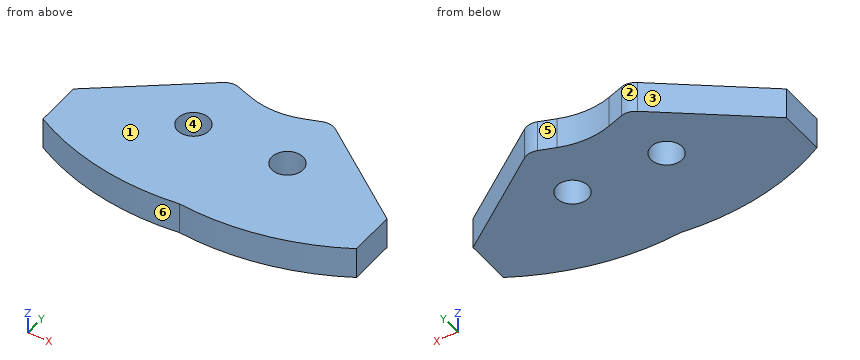
from build123d import *

# Parameters (mm, degrees)
SZKIC1_R                    = 5
DODANIE_WYCI_GNI_CIE1_DEPTH = 10


with BuildPart() as part:
    # Szkic1 → Dodanie-wyciągnięcie1 (new body)
    with BuildSketch(Plane.XY):
        with BuildLine():
            Line((0, 10), (0, 25))
            Line((0, 25), (31.999991312, 49.000008999))
            ThreePointArc((31.999991312, 49.000008999), (34.24374996, 49.942489803), (36.666669828, 49.714055442))
            Line((36.666669828, 49.714055442), (41.666653651, 47.946291102))
            ThreePointArc((41.666653651, 47.946291102), (50, 46.51651254), (58.333346349, 47.946291102))
            Line((58.333346349, 47.946291102), (63.333330172, 49.714055442))
            ThreePointArc((63.333330172, 49.714055442), (65.75625004, 49.942489803), (68.000008688, 49.000008999))
            Line((68.000008688, 49.000008999), (100, 25))
            Line((100, 25), (100, 10))
            ThreePointArc((100, 10), (75.784613824, 1.076930879), (50, 0))
            ThreePointArc((50, 0), (24.215386176, 1.076930879), (0, 10))
        make_face()
        with Locations((35, 30)):
            Circle(SZKIC1_R, mode=Mode.SUBTRACT)
        with Locations(Location((65, 30, 0), (0, 0, 180))):
            Circle(SZKIC1_R, mode=Mode.SUBTRACT)
    extrude(amount=DODANIE_WYCI_GNI_CIE1_DEPTH)


solid = part.part
Here's how the part is built. I have some questions about the finished solid (model axes, mm). Face numbers are marked on the shaded views. A direction names the side the tool comes from. Round coordinates to 2 decimals unless told otherwise and drop trailing zeros. Write each loop counter-clockwise with the first axis right and the second up, starting at its lowest first coordinate (ties: lowest second). Pieces come first, ordered by that corner, then holes. Notation, with made-up numbers: (9.5, 4) -> (26.5, 4) arc R35 ccw to (26.5, 40) -> close; hole circle Ø6 at (12.25, -30). An arc over 180 degrees is marked (long way). One line per item, written item: value.
1) Suppose I cut it at A-A on x = 38. List the corners of the cut face in (y, z) for me.
Filled sheet:
outline: (-0.5, 0) -> (26, 0) -> (26, 10) -> (-0.5, 10) -> close; (34, 0) -> (49.24, 0) -> (49.24, 10) -> (34, 10) -> close
2) Suppose I cut it at B-B on z = 4.75. List the corners of the cut face in (x, y) for me, plus the area to 3 significant figures.
Filled sheet:
outline: (0, 10) arc R83.23 ccw to (50, 0) arc R83.23 ccw to (100, 10) -> (100, 25) -> (68, 49) arc R5 ccw to (63.33, 49.71) -> (58.33, 47.95) arc R25 cw to (41.67, 47.95) -> (36.67, 49.71) arc R5 ccw to (32, 49) -> (0, 25) -> close; hole circle Ø10 at (35, 30); hole circle Ø10 at (65, 30)
area: 3,720 mm2
3) Suppose I cut it at D-D on x = 87.5. List the corners of the cut face in (y, z) for me (3 decimals).
Filled sheet:
outline: (4.325, 0) -> (34.375, 0) -> (34.375, 10) -> (4.325, 10) -> close
4) For the marked faces 5 and 6, which set-ups out of +Z, -Z, +X, -X, +Y, -Y let a thin tool reach every point of the face, with its end or its side?
Filled sheet:
face 5: +Z, -Z, +Y
face 6: +Z, -Z, -Y
5) I'm going to push flat-ended pins straight in: pin 1 Ø2 at (x, z) = (20, 2) entering from -Y; pin 2 Ø2 at (x, z) = (46, 3.5) entering from -Y. Where does each tip first touch, or does it pass through?
Filled sheet:
pin 1: stops at y = 1.79
pin 2: stops at y = -0.42
6) Suppose I cut it at C-C on y = 30. List the corners of the cut face in (x, z) for me, plus the area to 3 significant figures.
Filled sheet:
outline: (6.67, 0) -> (30, 0) -> (30, 10) -> (6.67, 10) -> close; (40, 0) -> (60, 0) -> (60, 10) -> (40, 10) -> close; (70, 0) -> (93.33, 0) -> (93.33, 10) -> (70, 10) -> close
area: 667 mm2
7) We'd pull the mould along X, two halves only. Please class the marked faces 1, 2, 3 and 4: released by +X, released by -X, zero draft, split by the parting line, or undercut.
Filled sheet:
face 1: zero draft
face 2: undercut
face 3: released by -X
face 4: undercut
8) If I drill on line 1 (Y direction, x = 39.5, z = 6); line 2 (Y direction, x = 37, z = 9); line 3 (Y direction, x = 81.5, z = 1.5) (3 decimals), over which ranges is the centre line in solid material (lowest first)? Write a range as [from, to].
Filled sheet:
line 1: y = [-0.53, 27.82], [32.18, 48.71]
line 2: y = [-0.46, 25.42], [34.58, 49.6]
line 3: y = [2.431, 38.875]
